```python
from build123d import *

# Parameters (mm, degrees)
SKETCH1_R                     = 20
SKETCH1_R_2                   = 4
BOSS_EXTRUDE1_DEPTH           = 22
SKETCH2_R                     = 17.5
SKETCH2_R_2                   = 4
BOSS_EXTRUDE2_DEPTH           = 2
SKETCH3_R                     = 17.5
SKETCH3_R_2                   = 11
BOSS_EXTRUDE3_DEPTH           = 2
SKETCH4_R                     = 20
SKETCH4_R_2                   = 11
BOSS_EXTRUDE4_DEPTH           = 13
F_4_0_4_DIAMETER_HOLE1_REACH  = 57.864
F_4_0_4_DIAMETER_HOLE1_BORE_R = 2
F_4_0_4_DIAMETER_HOLE2_REACH  = 57.96
F_4_0_4_DIAMETER_HOLE2_BORE_R = 2


with BuildPart() as part:
    # Sketch1 → Boss-Extrude1 (new body)
    with BuildSketch(Plane(origin=(0, 0, 0), x_dir=(1, 0, 0), z_dir=(0, 1, 0))):
        with Locations(Location((0, 0, 0), (0, 0, 270))):
            Circle(SKETCH1_R)
        with Locations(Location((0, 0, 0), (0, 0, 270))):
            Circle(SKETCH1_R_2, mode=Mode.SUBTRACT)
    extrude(amount=BOSS_EXTRUDE1_DEPTH)

    # Sketch2 → Boss-Extrude2 (add)
    with BuildSketch(Plane(origin=(0, 22, 0), x_dir=(1, 0, 0), z_dir=(0, 1, 0))):
        with Locations(Location((0, 0, 0), (0, 0, 270))):
            Circle(SKETCH2_R)
        with Locations(Location((0, 0, 0), (0, 0, 270))):
            Circle(SKETCH2_R_2, mode=Mode.SUBTRACT)
    extrude(amount=BOSS_EXTRUDE2_DEPTH)

    # Sketch3 → Boss-Extrude3 (add)
    with BuildSketch(Plane(origin=(0, 24, 0), x_dir=(1, 0, 0), z_dir=(0, 1, 0))):
        with Locations(Location((0, 0, 0), (0, 0, 270))):
            Circle(SKETCH3_R)
        with Locations(Location((0, 0, 0), (0, 0, 270))):
            Circle(SKETCH3_R_2, mode=Mode.SUBTRACT)
    extrude(amount=BOSS_EXTRUDE3_DEPTH)

    # Sketch4 → Boss-Extrude4 (add)
    with BuildSketch(Plane(origin=(0, 26, 0), x_dir=(1, 0, 0), z_dir=(0, 1, 0))):
        with Locations(Location((0, 0, 0), (0, 0, 270))):
            Circle(SKETCH4_R)
        with Locations(Location((0, 0, 0), (0, 0, 270))):
            Circle(SKETCH4_R_2, mode=Mode.SUBTRACT)
    extrude(amount=BOSS_EXTRUDE4_DEPTH)

    # Ø4.0 (4) Diameter Hole1 bore (on position points) → Ø4.0 (4) Diameter Hole1 (cut, up to next)
    with BuildSketch(Plane(origin=(16.590996999, 10.532581899, -11.168653391), x_dir=(0.55843266957, 0, 0.829549849953), z_dir=(0.829549849953, 0, -0.55843266957)), mode=Mode.PRIVATE) as f_4_0_4_diameter_hole1_sk1:
        Circle(F_4_0_4_DIAMETER_HOLE1_BORE_R)
    f_4_0_4_diameter_hole1_tool1 = extrude(f_4_0_4_diameter_hole1_sk1.sketch, amount=-F_4_0_4_DIAMETER_HOLE1_REACH, mode=Mode.PRIVATE) & part.part
    add(f_4_0_4_diameter_hole1_tool1.solids().sort_by_distance((16.590997, 10.532582, -11.168653))[0], mode=Mode.SUBTRACT)

    # Ø4.0 (4) Diameter Hole2 bore (on position points) → Ø4.0 (4) Diameter Hole2 (cut, up to next)
    with BuildSketch(Plane(origin=(-3.052461352, 31.918352454, -19.765689457), x_dir=(-0.98828447283, 0, 0.152623067601), z_dir=(-0.152623067601, 0, -0.98828447283)), mode=Mode.PRIVATE) as f_4_0_4_diameter_hole2_sk1:
        Circle(F_4_0_4_DIAMETER_HOLE2_BORE_R)
    f_4_0_4_diameter_hole2_tool1 = extrude(f_4_0_4_diameter_hole2_sk1.sketch, amount=-F_4_0_4_DIAMETER_HOLE2_REACH, mode=Mode.PRIVATE) & part.part
    add(f_4_0_4_diameter_hole2_tool1.solids().sort_by_distance((-3.052461, 31.918352, -19.765689))[0], mode=Mode.SUBTRACT)


solid = part.part
```
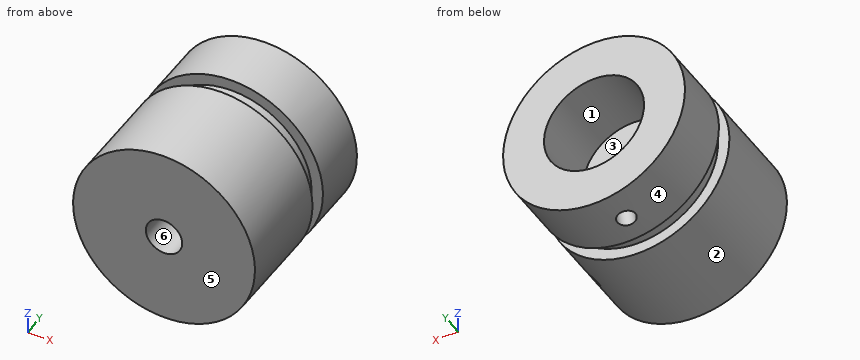
CAD build for the part. Positions are in the model's coordinates, mm. Face numbers are marked on the shaded views. A direction names the side the tool comes from. Give positions to 0.01 mm unless a question says otherwise; leave off trailing zeros. Write each loop counter-clockwise with the first axis right and the second up, starting at its lowest first coordinate (ties: lowest second). Pieces come first, ordered by that corner, then holes. Notation, with made-up numbers: M 25.25,54 L 45.25,54 A23 ccw 45.25,77 Z; hole C 32,44.5 d5. An arc over 180 degrees is marked long. Return JSON: item names as keys, results as strings. Group by question number.
(1) Mould opens along Z. For the marked faces 3, 4, 5 and 6 say: pulls with the +Z half, pulls with the -Z half, needs draft (parallel to the pull), parting line crosses it, or undercut.
(2) Flat gauge pins, fed straight in: pin 1 Ø3 at (x, y) = (-11.5, 24) entering from +Z; pin 2 Ø13 at (x, z) = (0, 0) entering from +Y; pin 3 Ø4 at (y, z) = (20, 8.5) entering from -X. Where does each tip first touch, or does it go through?
(3) Band-saw the part on D-D (y = 37.5). Give the cut face in (x, z), and give its area (3 significant figures).
(4) Band-saw the part on B-B (x = -6.5). Give the cut face in (y, z).
(5) Band-saw the part on A-A (y = 23). Give the cut face in (x, z).
(6) Band-saw the part on C-C (z = 16). Give the cut face in (x, y), and give its area (3 significant figures).
(7) Drill centre lines: L1, parallel to X at y = 18.75, z = 0; L2, parallel to Y at x = 17, z = 8.5; L3, parallel to X at y = 31, z = 0. Where is each one in solid material? Low to high. Write a range as [from, to].
(8) 3-axis set-ups, long thin cutter, end or side, ignore diameter. For the marked faces 1 and 2: which of +Z, -Z, +X, -X, +Y, -Y reach the whole face in a straight line?
Entries:
{
 "1": {"face 3": "undercut", "face 4": "parting line crosses it", "face 5": "needs draft", "face 6": "undercut"},
 "2": {"pin 1": "stops at z = 14.36", "pin 2": "stops at y = 24", "pin 3": "stops at x = -18.91"},
 "3": {"outline": "C 0,0 d40; hole C 0,0 d22", "area": "877 mm^2"},
 "4": {"outline": "M 0,-18.91 L 22,-18.91 L 22,-16.25 L 26,-16.25 L 26,-18.91 L 39,-18.91 L 39,-8.87 L 24,-8.87 L 24,8.87 L 39,8.87 L 39,18.91 L 26,18.91 L 26,16.25 L 22,16.25 L 22,18.91 L 0,18.91 Z"},
 "5": {"outline": "C 0,0 d35; hole C 0,0 d8"},
 "6": {"outline": "M -12,0 L 12,0 L 12,22 L 7.09,22 L 7.09,26 L 12,26 L 12,39 L -12,39 L -12,26 L -7.09,26 L -7.09,22 L -12,22 Z", "area": "897 mm^2"},
 "7": {"L1": "x = [-20, -4], [4, 20]", "L2": "y = [0, 22], [26, 39]", "L3": "x = [-20, -11], [11, 20]"},
 "8": {"face 1": "+Y", "face 2": "+Y, -Y"}
}
